from build123d import *

# Parameters (mm, degrees)
SKETCH2_W           = 65
SKETCH2_H           = 52
SKETCH2_R           = 1.5
BOSS_EXTRUDE1_DEPTH = 3
FILLET1_R           = 3
CUT_EXTRUDE1_START  = -10
SKETCH3_R           = 1.5
CUT_EXTRUDE1_DEPTH  = 10
SKETCH4_R           = 1.5
CUT_EXTRUDE2_DEPTH  = 10
FILLET2_R           = 3


with BuildPart() as part:
    # Sketch2 → Boss-Extrude1 (new body)
    with BuildSketch(Plane(origin=(0, 0, 0), x_dir=(1, 0, 0), z_dir=(0, 1, 0))):
        with Locations((-5, 0)):
            Rectangle(SKETCH2_W, SKETCH2_H)
        with Locations(Location((-24.875, 22.45, 0), (0, 0, 270))):
            Circle(SKETCH2_R, mode=Mode.SUBTRACT)
        with Locations(Location((24.875, 22.45, 0), (0, 0, 270))):
            Circle(SKETCH2_R, mode=Mode.SUBTRACT)
        with Locations(Location((24.875, -22.45, 0), (0, 0, 270))):
            Circle(SKETCH2_R, mode=Mode.SUBTRACT)
        with Locations(Location((-24.875, -22.45, 0), (0, 0, 270))):
            Circle(SKETCH2_R, mode=Mode.SUBTRACT)
    extrude(amount=BOSS_EXTRUDE1_DEPTH)

    # Fillet1
    fillet1_edges = [part.edges().sort_by_distance(p)[0] for p in [
        (-37.5, 1.5, 26),
        (-37.5, 1.5, -26),
        (27.5, 1.5, -26),
        (27.5, 1.5, 26),
    ]]
    fillet(fillet1_edges, radius=FILLET1_R)

    # Sketch3 → Cut-Extrude1 (cut)
    with BuildSketch(Plane(origin=(0, 3, 0), x_dir=(1, 0, 0), z_dir=(0, 1, 0)).offset(CUT_EXTRUDE1_START)):
        with Locations(Location((24.875, 22.45, 0), (0, 0, 270))):
            Circle(SKETCH3_R)
        with Locations(Location((-5.125, 22.45, 0), (0, 0, 270))):
            Circle(SKETCH3_R)
        with Locations(Location((-5.125, -22.45, 0), (0, 0, 270))):
            Circle(SKETCH3_R)
        with Locations(Location((24.875, -22.45, 0), (0, 0, 270))):
            Circle(SKETCH3_R)
    extrude(amount=CUT_EXTRUDE1_DEPTH, mode=Mode.SUBTRACT)

    # Sketch4 → Cut-Extrude2 (cut)
    with BuildSketch(Plane(origin=(0, 3, 0), x_dir=(1, 0, 0), z_dir=(0, 1, 0))):
        with BuildLine():
            Line((-9.9, -26), (-9.9, 0))
            Line((-9.9, 0), (-9.9, 26))
            Line((-9.9, 26), (-34.5, 26))
            ThreePointArc((-34.5, 26), (-36.621320344, 25.121320344), (-37.5, 23))
            Line((-37.5, 23), (-37.5, -23))
            ThreePointArc((-37.5, -23), (-36.621320344, -25.121320344), (-34.5, -26))
            Line((-34.5, -26), (-9.9, -26))
        make_face()
        with Locations((-24.875, -22.45)):
            Circle(SKETCH4_R, mode=Mode.SUBTRACT)
        with Locations((-24.875, 22.45)):
            Circle(SKETCH4_R, mode=Mode.SUBTRACT)
    extrude(amount=-CUT_EXTRUDE2_DEPTH, mode=Mode.SUBTRACT)

    # Fillet2
    fillet2_edges = [part.edges().sort_by_distance(p)[0] for p in [
        (-9.9, 1.5, -26),
        (-9.9, 1.5, 26),
    ]]
    fillet(fillet2_edges, radius=FILLET2_R)


solid = part.part
Geometry: final body of the model. Coordinates: model frame, mm. Coordinates: 2 decimals unless noted, no trailing zeros. Order: outer loops, then holes, each group sorted by start corner. A loop starts at its lowest first (then second) coordinate and runs counter-clockwise, first axis right, second up. Notation, with made-up numbers: M 85,-36 L 103,-36 A20 ccw 103,-31 Z; hole C 35.5,-27 d4. An arc over 180 degrees is marked long. One line per question, with ' | ' between items. Start each with the question number.
Item 1: Ray query, probe 1 along X at (y, z) = (2.15, -22.45) (3 decimals); probe 2 along Z at (x, y) = (-6.5, 0.25); probe 3 along Z at (x, y) = (26, 1.8). Return the intervals inside material, ascending. Write a range as [from, to].
Item 2: Cut plane B-B, the plane y = 2.4. Return the cut outline in (x, z) (3 decimals), then the cut area to 3 significant figures.
Item 3: Draft query along X for faces 1 (the flat face through (9, 3, 0)), 2 (the cylindrical face through (26.36, 1.48, -22.65)), 3 (the flat face through (-9.9, 2, 0)). Return one class per face: released by +X, released by -X, zero draft, split by the parting line, or undercut.
Item 4: Pin query (flat end, axial travel): pin 1 Ø2.5 at (x, z) = (24.875, -22.45) entering from -Y. Return the tip coordinate at first contact, or that it passes through.
Item 5: Cut plane A-A, the plane z = -22.45. Return the cut outline in (x, y) (3 decimals).
A:
1) probe 1: x = [-9.9, -6.625], [-3.625, 23.375], [26.375, 27.5] | probe 2: z = [-26, -23.05], [-21.85, 21.85], [23.05, 26] | probe 3: z = [-25.6, -23.44], [-21.46, 21.46], [23.44, 25.6]
2) outline: M -9.9,-23 A3 ccw -6.9,-26 L 24.5,-26 A3 ccw 27.5,-23 L 27.5,23 A3 ccw 24.5,26 L -6.9,26 A3 ccw -9.9,23 Z; hole C -5.125,-22.45 d3; hole C -5.125,22.45 d3; hole C 24.875,-22.45 d3; hole C 24.875,22.45 d3 | area: 1,910 mm2
3) face 1: zero draft | face 2: undercut | face 3: released by -X
4) pin 1: passes through
5) outline: M -9.9,0 L -6.625,0 L -6.625,3 L -9.9,3 Z; M -3.625,0 L 23.375,0 L 23.375,3 L -3.625,3 Z; M 26.375,0 L 27.5,0 L 27.5,3 L 26.375,3 Z
